```python
from build123d import *

# Parameters (mm, degrees)
EXTRUDE_1_DEPTH        = 98
HOLE_WIZARD_M5_1_D     = 4.2
HOLE_WIZARD_M5_1_DEPTH = 14
HOLE_WIZARD_M5_1_TIP   = 1.2618073
HOLE_WIZARD_M5_2_D     = 4.2
HOLE_WIZARD_M5_2_DEPTH = 14
HOLE_WIZARD_M5_2_TIP   = 1.2618073


with BuildPart() as part:
    # 草图1 → 凸台-拉伸1 (new body)
    with BuildSketch(Plane.XY):
        Polygon((0, 0), (0, 128), (-5, 128), (-5, 5), (-20, 5), (-20, 0), align=None)
    extrude(amount=EXTRUDE_1_DEPTH)

    # M5 螺纹孔1
    with Locations(Plane(origin=(0, 5, 0), x_dir=(1, 0, 0), z_dir=(0, 1, 0))):
        with Locations((-12.5, -24), (-12.5, -74)):
            Hole(HOLE_WIZARD_M5_1_D / 2, depth=HOLE_WIZARD_M5_1_DEPTH)
            with Locations((0, 0, -(HOLE_WIZARD_M5_1_DEPTH + HOLE_WIZARD_M5_1_TIP / 2))):  # 118° drill point
                Cone(0, HOLE_WIZARD_M5_1_D / 2, HOLE_WIZARD_M5_1_TIP, mode=Mode.SUBTRACT)

    # M5 螺纹孔2
    with Locations(Plane.ZY.offset(5)):
        with Locations((24, 58), (49, 58), (74, 58), (74, 83), (74, 108), (49, 108), (24, 108), (24, 83), (49, 83)):
            Hole(HOLE_WIZARD_M5_2_D / 2, depth=HOLE_WIZARD_M5_2_DEPTH)
            with Locations((0, 0, -(HOLE_WIZARD_M5_2_DEPTH + HOLE_WIZARD_M5_2_TIP / 2))):  # 118° drill point
                Cone(0, HOLE_WIZARD_M5_2_D / 2, HOLE_WIZARD_M5_2_TIP, mode=Mode.SUBTRACT)


solid = part.part
```
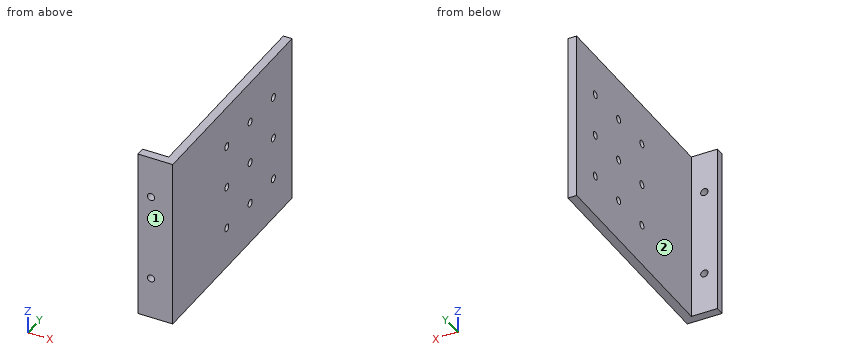
Could you check a few things on this model? Use its own coordinates, in mm. Face numbers are marked on the shaded views. A direction names the side the tool comes from. Coordinates: 2 decimals unless noted, no trailing zeros. Loops run counter-clockwise (first coordinate to the right, second up) from the corner with the lowest first, then second, coordinate; pieces in that order, holes last. Notation, with made-up numbers: M 67.5,78.5 L 78.5,78.5 A16 cw 78.5,82.5 Z; hole C 29.5,6 d2. An arc over 180 degrees is marked long. Put each result on its own line as item: value. Start each with the question number.
(1) Will these pins go through, and if not, where does the flat tip stop? P1, Ø2, axis at x = -10.5, z = 62.5, coming from the +Y side; P2, Ø1, axis at y = 57.5, z = 78, coming from the -X side.
(2) Suppose I cut it at D-D on z = 24. Please give me the cut outline in (x, y), then the cut area to 3 significant figures.
(3) Suppose I cut it at C-C on y = 83. Please give me the cut outline in (x, z), then the cut area to 3 significant figures.
(4) Suppose I cut it at B-B on z = 49. Please give me the cut outline in (x, y), then the cut area to 3 significant figures.
(5) For the marked faces 1 and 2, which set-ups out of +Z, -Z, +X, -X, +Y, -Y let a thin tool reach every point of the face, with its end or its side?
(6) I need wall thicknesses on line 1 (Y direction, x = -1.2, z = 74); line 2 (X direction, y = 1.9, z = 74); line 3 (X direction, y = 36.5, z = 34). Which ranges of each line are inside material? Lowest first, please. Write a range as from..to.
(7) Suppose I cut it at A-A on x = -12.5. Please give me the cut outline in (y, z), then the cut area to 3 significant figures.
Solutions:
1. P1: stops at y = 5
1. P2: stops at x = -5
2. outline: M -20,0 L -14.6,0 L -14.6,5 L -20,5 Z; M -10.4,0 L 0,0 L 0,55.9 L -5,55.9 L -5,5 L -10.4,5 Z; M -5,60.1 L 0,60.1 L 0,80.9 L -5,80.9 Z; M -5,85.1 L 0,85.1 L 0,105.9 L -5,105.9 Z; M -5,110.1 L 0,110.1 L 0,128 L -5,128 Z
2. area: 631 mm2
3. outline: M -5,0 L 0,0 L 0,21.9 L -5,21.9 Z; M -5,26.1 L 0,26.1 L 0,46.9 L -5,46.9 Z; M -5,51.1 L 0,51.1 L 0,71.9 L -5,71.9 Z; M -5,76.1 L 0,76.1 L 0,98 L -5,98 Z
3. area: 427 mm2
4. outline: M -20,0 L 0,0 L 0,55.9 L -5,55.9 L -5,5 L -20,5 Z; M -5,60.1 L 0,60.1 L 0,80.9 L -5,80.9 Z; M -5,85.1 L 0,85.1 L 0,105.9 L -5,105.9 Z; M -5,110.1 L 0,110.1 L 0,128 L -5,128 Z
4. area: 652 mm2
5. face 1: +Z, -Z, +X, -X, -Y
5. face 2: +Z, -Z, -X, +Y
6. line 1: y = 0..55.9, 60.1..80.9, 85.1..105.9, 110.1..128
6. line 2: x = -20..-14.6, -10.4..0
6. line 3: x = -5..0
7. outline: M 0,0 L 5,0 L 5,21.9 L 0,21.9 Z; M 0,26.1 L 5,26.1 L 5,71.9 L 0,71.9 Z; M 0,76.1 L 5,76.1 L 5,98 L 0,98 Z
7. area: 448 mm2
